```python
from build123d import *

# Parameters (mm, degrees)
SKETCH1_R               = 3
BOSS_EXTRUDE1_DEPTH     = 12
SKETCH2_R               = 1.095
CUT_EXTRUDE1_DEPTH      = 7
SKETCH3_R               = 1
CUT_EXTRUDE2_DEPTH      = 0.7
CUT_EXTRUDE3_REACH      = 15.599
CUT_EXTRUDE3_END_RADIUS = 1.095
SKETCH4_R               = 0.5
SKETCH5_R               = 0.9975
CUT_EXTRUDE4_DEPTH      = 3


with BuildPart() as part:
    # Sketch1 → Boss-Extrude1 (new body)
    with BuildSketch(Plane(origin=(0, 0, 0), x_dir=(0, 0, -1), z_dir=(1, 0, 0))):
        Circle(SKETCH1_R)
    extrude(amount=BOSS_EXTRUDE1_DEPTH)

    # Sketch2 → Cut-Extrude1 (cut)
    with BuildSketch(Plane(origin=(0, 0, 0), x_dir=(0, 0, -1), z_dir=(1, 0, 0))):
        Circle(SKETCH2_R)
    extrude(amount=CUT_EXTRUDE1_DEPTH, mode=Mode.SUBTRACT)

    # Sketch3 → Cut-Extrude2 (cut)
    with BuildSketch(Plane(origin=(0, 3, 0), x_dir=(1, 0, 0), z_dir=(0, 1, 0))):
        with Locations(Location((3, 0, 0), (0, 0, 270))):
            Circle(SKETCH3_R)
    extrude(amount=-CUT_EXTRUDE2_DEPTH, mode=Mode.SUBTRACT)

    # Cut-Extrude3: up to this cylinder (the profile starts outside it)
    cut_extrude3_end = Plane(origin=(3, 0, 0), z_dir=(-1, 0, 0)) * Cylinder(CUT_EXTRUDE3_END_RADIUS, 34.388, mode=Mode.PRIVATE)
    # Sketch4 → Cut-Extrude3 (cut, up to the surface)
    with BuildSketch(Plane(origin=(0, 2.65, 0), x_dir=(1, 0, 0), z_dir=(0, 1, 0)), mode=Mode.PRIVATE) as cut_extrude3_sk1:
        with Locations(Location((3, 0, 0), (0, 0, 270))):
            Circle(SKETCH4_R)
    cut_extrude3_tool1 = extrude(cut_extrude3_sk1.sketch, amount=-CUT_EXTRUDE3_REACH, mode=Mode.PRIVATE) - cut_extrude3_end
    add(cut_extrude3_tool1.solids().sort_by_distance((3, 2.65, 0))[0], mode=Mode.SUBTRACT)

    # Sketch5 → Cut-Extrude4 (cut)
    with BuildSketch(Plane(origin=(12, 0, 0), x_dir=(0, 0, -1), z_dir=(1, 0, 0))):
        Circle(SKETCH5_R)
    extrude(amount=-CUT_EXTRUDE4_DEPTH, mode=Mode.SUBTRACT)


solid = part.part
```
Source: CAD feature listing. Evaluate the final solid. Frame: model axes, mm. A direction names the side the tool comes from. Give positions to 0.01 mm unless a question says otherwise; leave off trailing zeros. Loops run counter-clockwise (first coordinate to the right, second up) from the corner with the lowest first, then second, coordinate; pieces in that order, holes last. Notation, with made-up numbers: (-6.5, 79.5) -> (32.5, 79.5) arc R19 cw to (32.5, 112.5) -> close; hole circle Ø6 at (55.25, 13). An arc over 180 degrees is marked (long way). Use a Markdown table: item, result. Add a question column.
(1) Section query A-A (z = 0). Output: boundary loops of the cut face in (x, y) (1 decimal).
(2) Ray query, line 1 (Y direction, x = 5.75, z = 0) (3 decimals); line 2 (Y direction, x = 10.95, z = 0); line 3 (Z direction, x = 3, y = 1.8). Return the intervals inside material, ascending.
(3) Section query D-D (x = 3). Output: boundary loops of the cut face in (y, z) (3 decimals), then the cut area to 3 significant figures.
(4) Pull-direction query (Y, two-part tool) for faces 1 (the face through (3.45, -0.97, -0.51)), 2 (the face through (5.92, -2.93, 0.65)), 3 (the face through (0, 0, -1.3)); classes: +Y half, -Y half, draft (parallel to the pull), parting line (faces both ways), or undercut.
(5) Access query for faces 4 (the face through (3, 1.6, -0.5)), 5 (the face through (7, 0, 0)), 6 (the face through (10.52, -0.61, 0.79)), 7 (the face through (12, 1, 1)). Directions: +Z, -Z, +X, -X, +Y, -Y. A direction counts if a zero-diameter tool reaches every point of the face in a straight line with its end or side. Return the directions, or none.
(6) Section query C-C (x = 6). Output: boundary loops of the cut face in (y, z) (3 decimals).
(7) Section query B-B (y = 0). Output: boundary loops of the cut face in (x, z) (1 decimal), then the cut area to 3 significant figures.
(8) First-contact query: pin 1 Ø1.5 at (x, z) = (3.5, 2) entering from -Y; pin 2 Ø0.7 at (y, z) = (0, -0.5) entering from -X; pin 3 Ø1 at (x, z) = (3.5, -0.5) entering from +Y. Flat tips, straight axial feed; report the tip coordinate or a pass-through.
Checked values:
| question | item | result |
|---|---|---|
| 1 | outline | (0, -3) -> (12, -3) -> (12, -1) -> (9, -1) -> (9, 1) -> (12, 1) -> (12, 3) -> (4, 3) -> (4, 2.3) -> (3.5, 2.3) -> (3.5, 1.1) -> (7, 1.1) -> (7, -1.1) -> (0, -1.1) -> close; (0, 1.1) -> (2.5, 1.1) -> (2.5, 2.3) -> (2, 2.3) -> (2, 3) -> (0, 3) -> close |
| 2 | line 1 | -3 to -1.095, 1.095 to 3 |
| 2 | line 2 | -3 to -1, 1 to 3 |
| 2 | line 3 | -2.4 to -0.5, 0.5 to 2.4 |
| 3 | outline | (0.974, -0.5) arc R1.095 cw (long way) to (0.974, 0.5) -> (2.3, 0.5) -> (2.3, 1) -> (2.828, 1) arc R3 ccw (long way) to (2.828, -1) -> (2.3, -1) -> (2.3, -0.5) -> close |
| 3 | area | 22.0 mm^2 |
| 4 | face 1 | undercut |
| 4 | face 2 | parting line |
| 4 | face 3 | draft |
| 5 | face 4 | +Y |
| 5 | face 5 | -X |
| 5 | face 6 | +X |
| 5 | face 7 | +Z, -Z, +X, +Y, -Y |
| 6 | outline | circle Ø6 at (0, 0); hole circle Ø2.19 at (0, 0) |
| 7 | outline | (0, -3) -> (12, -3) -> (12, -1) -> (9, -1) -> (9, 1) -> (12, 1) -> (12, 3) -> (0, 3) -> (0, 1.1) -> (7, 1.1) -> (7, -1.1) -> (0, -1.1) -> close |
| 7 | area | 50.7 mm^2 |
| 8 | pin 1 | y = -2.73 |
| 8 | pin 2 | x = 7 |
| 8 | pin 3 | y = 2.99 |
